Check sheet for the modelled part. Datum: model origin and axes. Units: mm. Face numbers are marked on the shaded views. A direction names the side the tool comes from. Round coordinates to 2 decimals unless told otherwise and drop trailing zeros. Write each loop counter-clockwise with the first axis right and the second up, starting at its lowest first coordinate (ties: lowest second). Pieces come first, ordered by that corner, then holes.
from build123d import *

# Parameters (mm, degrees)
CHAMFER1_SIZE      = 1.35
FILLET1_R          = 0.25
CHAMFER2_SIZE      = 0.381
SKETCH2_W          = 16
SKETCH2_H          = 8.508
CUT_EXTRUDE1_DEPTH = 13
SKETCH3_W          = 1.016
SKETCH3_H          = 8
CUT_EXTRUDE2_DEPTH = 8
SCALE2_SCALE       = 1.001


with BuildPart() as part:
    # Sketch1 → Revolve1 (revolve)
    with BuildSketch(Plane.XY, mode=Mode.PRIVATE) as revolve1_sk:
        Polygon((3.25, 0), (3.25, 2), (6, 2), (6, 12), (8, 12), (8, 0), align=None)
    revolve(revolve1_sk.sketch.rotate(Axis((0, 0, 0), (0, 1, 0)), 90), axis=Axis((0, 0, 0), (0, 1, 0)))  # turned: the seam where the file's is

    # Chamfer1
    chamfer1_edges = [part.edges().sort_by_distance(p)[0] for p in [
        (0, 2, 3.25),
    ]]
    chamfer(chamfer1_edges, length=CHAMFER1_SIZE)

    # Fillet1
    fillet1_edges = [part.edges().sort_by_distance(p)[0] for p in [
        (0, 2, 6),
    ]]
    fillet(fillet1_edges, radius=FILLET1_R)

    # Chamfer2
    chamfer2_edges = [part.edges().sort_by_distance(p)[0] for p in [
        (0, 0, 8),
        (0, 12, 8),
        (0, 12, 6),
    ]]
    chamfer(chamfer2_edges, length=CHAMFER2_SIZE)

    # Sketch2 → Cut-Extrude1 (cut, through all)
    with BuildSketch(Plane(origin=(0, 0, 0), x_dir=(1, 0, 0), z_dir=(0, 1, 0))):
        with Locations((0, 3.746)):
            Rectangle(SKETCH2_W, SKETCH2_H)
    extrude(amount=CUT_EXTRUDE1_DEPTH, mode=Mode.SUBTRACT)

    # Sketch3 → Cut-Extrude2 (cut)
    with BuildSketch(Plane(origin=(0, 0, 0), x_dir=(1, 0, 0), z_dir=(0, 1, 0))):
        with Locations((0, -4)):
            Rectangle(SKETCH3_W, SKETCH3_H)
    extrude(amount=CUT_EXTRUDE2_DEPTH, mode=Mode.SUBTRACT)


with BuildPart() as part_1:
    # Scale2: scaled about (0, 0, 0)
    add(part.part.scale(SCALE2_SCALE))


solid = part_1.part
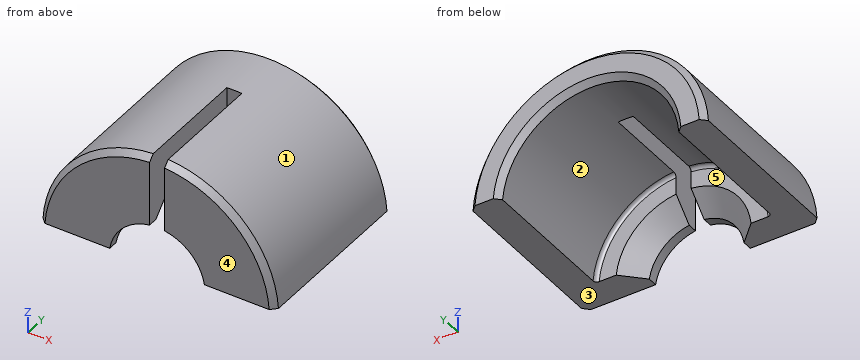
1. Sectioned sample at B-B, the plane x = 0. Enter the section's corners in (y, z).
2. Set-up check for the marked faces 4 and 5: record each of +Z, -Z, +X, -X, +Y, -Y from which the full face is reachable in a straight line by a thin tool's end or side.
3. Scan lines: line 1 along Z through (x, y) = (0.5, 8.5); line 2 along X through (y, z) = (4.5, 2.25); line 3 along X through (y, z) = (6.5, 6.5). Record each from-to range of solid material in increasing order.
4. Sectioned sample at C-C, the plane y = 11. Enter the section's corners in (x, z).
5. Sectioned sample at A-A, the plane y = 1.5. Enter the section's corners in (x, z), plus the area to 3 significant figures.
6. Go/stop test with flat-tipped pins: pin 1 (2.5 mm diameter, centred on y = 2, z = 6.5, fed in from -X); pin 2 (1.5 mm diameter, centred on x = 3, y = 8.5, fed in from +Z); pin 3 (2.5 mm diameter, centred on y = 5, z = 5.5, fed in from +X). Record where each tip stops, or that it passes through.
7. Release check for a two-part mould opening along X. For the marked faces 1, 2 and 3 record: released by +X, released by -X, zero draft, split by the parting line, or undercut.
Computed values:
1. outline: (8.01, 6.01) - (11.63, 6.01) - (12.01, 6.39) - (12.01, 7.63) - (11.63, 8.01) - (8.01, 8.01) - close
2. face 4: +Z, -Z, +X, -X, -Y
2. face 5: -Z, +Y
3. line 1: z = 5.99 to 7.99
3. line 2: x = -7.69 to -5.57, 5.57 to 7.69
3. line 3: x = -4.68 to -0.51, 0.51 to 4.68
4. outline: (-7.99, 0.51) - (-5.98, 0.51) arc R6.01 cw to (5.98, 0.51) - (7.99, 0.51) arc R8.01 ccw to start
5. outline: (-7.99, 0.51) - (-4.07, 0.51) arc R4.1 cw to (-0.51, 4.07) - (-0.51, 7.99) arc R8.01 ccw to start; (0.51, 4.07) arc R4.1 cw to (4.07, 0.51) - (7.99, 0.51) arc R8.01 ccw to (0.51, 7.99) - close
5. area: 66.3 mm2
6. pin 1: stops at x = -6.05
6. pin 2: stops at z = 7.69
6. pin 3: stops at x = 6.79
7. face 1: split by the parting line
7. face 2: undercut
7. face 3: zero draft
